```python
from build123d import *

# Parameters (mm, degrees)
BASEHEAD_DEPTH = 26


with BuildPart() as part:
    # HeadSke → BaseHead (new body)
    with BuildSketch(Plane(origin=(0, 0, 0), x_dir=(0, 0, -1), z_dir=(1, 0, 0))):
        Polygon((32.5, 18.763883749), (32.5, -18.763883749), (0, -37.527767497), (-32.5, -18.763883749), (-32.5, 18.763883749), (0, 37.527767497), align=None)
    extrude(amount=BASEHEAD_DEPTH)

    # BodySke → BaseBody (revolve)
    with BuildSketch(Plane.XY, mode=Mode.PRIVATE) as basebody_sk:
        Polygon((0, 0), (226, 0), (226, 18.533), (223.533, 21), (0, 21), align=None)
    revolve(basebody_sk.sketch.rotate(Axis((0, 0, 0), (1, 0, 0)), 90), axis=Axis((0, 0, 0), (1, 0, 0)))

    # Sketch3 → HeadChamfer (revolve, cut)
    with BuildSketch(Plane(origin=(0, 0, 0), x_dir=(1, 0, 0), z_dir=(0, 1, 0))):
        Polygon((-8.125, 18.427087189), (8.125, 46.572912811), (-13.525635095, 59.072912811), (-29.775635095, 30.927087189), align=None)
    revolve(axis=Axis((0, 0, 0), (1, 0, 0)), mode=Mode.SUBTRACT)

    # BearingSke → BearingFace (revolve, cut)
    with BuildSketch(Plane.XY, mode=Mode.PRIVATE) as bearingface_sk:
        Polygon((26, 30.3), (25, 32.032050808), (25, 37.527767497), (26, 37.527767497), align=None)
    revolve(bearingface_sk.sketch.rotate(Axis((0, 0, 0), (1, 0, 0)), 90), axis=Axis((0, 0, 0), (1, 0, 0)), mode=Mode.SUBTRACT)


solid = part.part
```
Geometry check sheet. Reference: the model listing, model coordinates, mm. A direction names the side the tool comes from. Give positions to 0.01 mm unless a question says otherwise; leave off trailing zeros. Write each loop counter-clockwise with the first axis right and the second up, starting at its lowest first coordinate (ties: lowest second). Pieces come first, ordered by that corner, then holes. Notation, with made-up numbers: (52.25, 68) -> (111.25, 68) arc R27 ccw to (111.25, 102) -> close; hole circle Ø11 at (7, -17). An arc over 180 degrees is marked (long way). Use one line per item in the form item = value.
Item 1: Access from +Z, -Z, +X, -X, +Y, -Y to the whole of each face (thin tool, end or side, straight path). Record for faces 1 (the flat face through (26, 7, 20)), 2 (the flat face through (12.3, -28, -16.5)).
Results list:
face_1 = +X
face_2 = -Z, +X, -X, -Y
Item 2: Depth check by flat-ended pin: pin 1 Ø1.5 at (x, y) = (43.5, -19.5) entering from +Z; pin 2 Ø10 at (x, z) = (120.5, 23.5) entering from -Y; pin 3 Ø2 at (x, y) = (110, -12) entering from +Z; pin 4 Ø5 at (x, z) = (196.5, 24.5) entering from +Y. Enter the tip coordinate at first touch or a pass-through.
Results list:
pin_1 = 9.46
pin_2 = -9.94
pin_3 = 17.89
pin_4 = through
Item 3: Sectioned sample at A-A on x = 99.5. Enter the section's corners in (y, z).
Results list:
outline = circle Ø42 at (0, 0)
Item 4: Scan lines: line 1 (Y direction, x = 36, z = 9.5); line 2 (X direction, y = -22, z = 15.5). Record each from-to range of solid material in increasing order.
Results list:
line_1 = -18.73 to 18.73
line_2 = 0 to 26
